Can you work these out from the model? Positions are in its coordinate system, mm. A direction names the side the tool comes from. Give positions to 0.01 mm unless a question says otherwise; leave off trailing zeros. Write item = value, one per line.
from build123d import *

# Parameters (mm, degrees)
SKETCH4_R          = 2
CUT_EXTRUDE1_DEPTH = 6
SKETCH5_R          = 1.5
CUT_EXTRUDE2_DEPTH = 159.778667329
SKETCH6_R          = 3.5
CUT_EXTRUDE3_DEPTH = 6.4


with BuildPart() as part:
    # Sketch3 (on Front Plane) → Revolve7 (revolve)
    with BuildSketch(Plane.XY, mode=Mode.PRIVATE) as revolve7_sk:
        with BuildLine():
            Line((-111, -28), (-101, -28))
            Line((-101, -28), (-101, -16.924568901))
            Line((-101, -16.924568901), (-109.95, -16.924568901))
            Line((-109.95, -16.924568901), (-109.95, -21.849137803))
            Line((-109.95, -21.849137803), (-112, -23.899137803))
            Line((-112, -23.899137803), (-112, -27))
            ThreePointArc((-112, -27), (-111.707106781, -27.707106781), (-111, -28))
        make_face()
    revolve(revolve7_sk.sketch.rotate(Axis((0, 0, 0), (0, 1, 0)), 270), axis=Axis((0, 0, 0), (0, 1, 0)))

    # Sketch4 → Cut-Extrude1 (cut)
    with BuildSketch(Plane(origin=(0, -16.924568901, 0), x_dir=(1, 0, 0), z_dir=(0, 1, 0))):
        with Locations(Location((0, 105.475, 0), (0, 0, 270))):
            Circle(SKETCH4_R)
        with Locations(Location((61.996649486, 85.331067482, 0), (0, 0, 270))):
            Circle(SKETCH4_R)
        with Locations(Location((100.312686056, 32.593567482, 0), (0, 0, 270))):
            Circle(SKETCH4_R)
        with Locations(Location((100.312686056, -32.593567482, 0), (0, 0, 270))):
            Circle(SKETCH4_R)
        with Locations(Location((61.996649486, -85.331067482, 0), (0, 0, 270))):
            Circle(SKETCH4_R)
        with Locations(Location((0, -105.475, 0), (0, 0, 270))):
            Circle(SKETCH4_R)
        with Locations(Location((-61.996649486, -85.331067482, 0), (0, 0, 270))):
            Circle(SKETCH4_R)
        with Locations(Location((-100.312686056, -32.593567482, 0), (0, 0, 270))):
            Circle(SKETCH4_R)
        with Locations(Location((-100.312686056, 32.593567482, 0), (0, 0, 270))):
            Circle(SKETCH4_R)
        with Locations(Location((-61.996649486, 85.331067482, 0), (0, 0, 270))):
            Circle(SKETCH4_R)
    extrude(amount=-CUT_EXTRUDE1_DEPTH, mode=Mode.SUBTRACT)

    # Sketch5 → Cut-Extrude2 (cut, through all)
    with BuildSketch(Plane(origin=(0, -16.924568901, 0), x_dir=(1, 0, 0), z_dir=(0, 1, 0))):
        with Locations(Location((-105.475, 0, 0), (0, 0, 270))):
            Circle(SKETCH5_R)
        with Locations(Location((-32.593567482, 100.312686056, 0), (0, 0, 270))):
            Circle(SKETCH5_R)
        with Locations(Location((85.331067482, 61.996649486, 0), (0, 0, 270))):
            Circle(SKETCH5_R)
        with Locations(Location((85.331067482, -61.996649486, 0), (0, 0, 270))):
            Circle(SKETCH5_R)
        with Locations(Location((-32.593567482, -100.312686056, 0), (0, 0, 270))):
            Circle(SKETCH5_R)
    extrude(amount=-CUT_EXTRUDE2_DEPTH, mode=Mode.SUBTRACT)

    # Sketch6 → Cut-Extrude3 (cut)
    with BuildSketch(Plane.XZ.offset(28)):
        with Locations(Location((-105.475, 0, 0), (0, 0, 270))):
            Circle(SKETCH6_R)
        with Locations(Location((-32.593567482, 100.312686056, 0), (0, 0, 270))):
            Circle(SKETCH6_R)
        with Locations(Location((85.331067482, 61.996649486, 0), (0, 0, 270))):
            Circle(SKETCH6_R)
        with Locations(Location((85.331067482, -61.996649486, 0), (0, 0, 270))):
            Circle(SKETCH6_R)
        with Locations(Location((-32.593567482, -100.312686056, 0), (0, 0, 270))):
            Circle(SKETCH6_R)
    extrude(amount=-CUT_EXTRUDE3_DEPTH, mode=Mode.SUBTRACT)


solid = part.part
Q1. We'd pull the mould along Z, two halves only. Please class faces 3 (the cylindrical face through (-34.723, -24.845, 103.09)), 4 (the cylindrical face through (-74.309, -19.421, 81.038)), 5 (the flat face through (89.1, -16.925, 48.4)): released by +Z, released by -Z, zero draft, split by the parting line, or undercut.
Output:
face_3 = undercut
face_4 = split by the parting line
face_5 = zero draft
Q2. For pin 1 (3 mm diameter, centred on x = -100.5, z = 31.5, fed in from +Y); pin 2 (1 mm diameter, centred on x = 44.5, y = -20, fed in from +Z); pin 3 (2 mm diameter, centred on x = -33, z = -101.5, fed in from -Y); pin 4 (1 mm diameter, centred on y = -19, z = 17, fed in from -X), each with a flat end and sliding along its axis, tell me the tip position at first contact or that it passes through.
Output:
pin_1 = -16.92
pin_2 = 100.76
pin_3 = -21.6
pin_4 = -108.7
Q3. Which directions (+Z, -Z, +X, -X, +Y, -Y) give clear straight access to the entire face, cutting with the end or side of a thin tool? Please do faces 1 (the flat face through (-105, -21.6, -2)), 2 (the flat face through (98.1, -28, 25.2)).
Output:
face_1 = -Y
face_2 = +Z, -Z, +X, -X, -Y
Q4. I need wall thicknesses on L1, parallel to Z at x = -61.5, y = -22.25; L2, parallel to Z at x = 2.5, y = -17.25; L3, parallel to X at y = -24.5, z = -22.5. Which ranges of each line are inside material? Lowest first, please.
Output:
L1 = -91.62 to -87.27, -83.39 to -80.12, 80.12 to 83.39, 87.27 to 91.62
L2 = -109.92 to -100.97, 100.97 to 109.92
L3 = -109.72 to -98.46, 98.46 to 109.72
Q5. Imagine slicing it at A-A, the plane y = -19.5. Give the number of separate pieces and of enclosed holes in the cut face, then the cut area to 3 significant figures.
Output:
separate_pieces = 1
enclosed_holes = 16
area = 5,770 mm2
